Geometry check sheet. Reference: the model listing, model coordinates, mm. Face numbers are marked on the shaded views. A direction names the side the tool comes from. Round coordinates to 2 decimals unless told otherwise and drop trailing zeros. Order: outer loops, then holes, each group sorted by start corner. A loop starts at its lowest first (then second) coordinate and runs counter-clockwise, first axis right, second up.
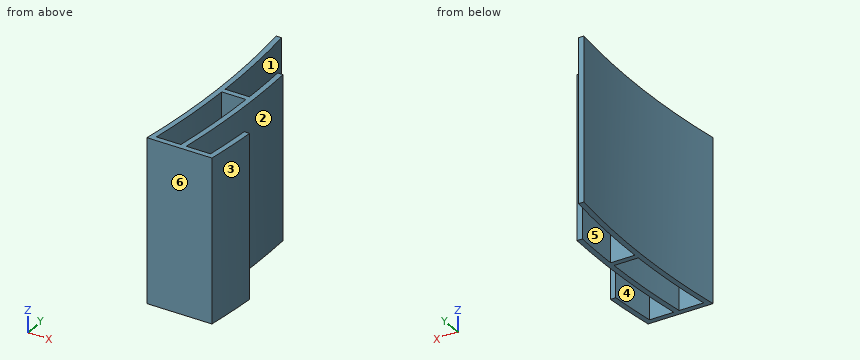
```python
from build123d import *

# Parameters (mm, degrees)
PAD_DEPTH = 60


with BuildPart() as part:
    # Sketch → Pad (new body)
    with BuildSketch(Plane.XY):
        with BuildLine():
            Line((2.414743, -35), (11.414743, -35))
            ThreePointArc((11.414743, -35), (11.263358, -26.246135), (10.865622, -17.5))
            Line((10.865622, -17.5), (12.865622, -17.5))
            ThreePointArc((11.335628, -72), (13.289566, -44.783378), (12.865622, -17.5))
            Line((11.335628, -72), (20.335628, -72))
            ThreePointArc((20.335628, -72), (21.198564, -63.260143), (21.822782, -54.5))
            Line((21.822782, -54.5), (23.822782, -54.5))
            ThreePointArc((22.11492, -74), (23.116177, -64.262903), (23.822782, -54.5))
            Line((22.11492, -74), (-2, -74))
            ThreePointArc((-2, -74), (0.416398, -36), (-2, 2))
            Line((-2, 2), (0.016131, 2))
            ThreePointArc((2.414743, -35), (1.783801, -16.463154), (0.016131, 2))
        make_face()
        with BuildLine():
            Line((2.414743, -37), (11.414743, -37))
            ThreePointArc((9.325722, -72), (10.863864, -54.529463), (11.414743, -37))
            Line((9.325722, -72), (0.263026, -72))
            ThreePointArc((0.263026, -72), (1.847307, -54.531257), (2.414743, -37))
        make_face(mode=Mode.SUBTRACT)
    extrude(amount=PAD_DEPTH)


solid = part.part
```
(1) Sectioned sample at B-B, the plane x = 4.5. Record the cut outline in (y, z).
Returned:
outline: (-74, 0) - (-72, 0) - (-72, 60) - (-74, 60) - close; (-37, 0) - (-35, 0) - (-35, 60) - (-37, 60) - close
(2) Material ranges on line 1 (Y direction, x = 9, z = 52); line 2 (Y direction, x = 14, z = 4.5); line 3 (X direction, y = -36, z = 15), recorded low to high.
Returned:
line 1: y = -74 to -72, -37 to -35
line 2: y = -74 to -72
line 3: x = 0.42 to 13.41
(3) Sectioned sample at A-A, the plane z = 37.5. Record the cut outline in (x, y), and give its area (3 significant figures).
Returned:
outline: (-2, -74) - (22.11, -74) arc R323.94 ccw to (23.82, -54.5) - (21.82, -54.5) arc R321.94 cw to (20.34, -72) - (11.34, -72) arc R313 ccw to (12.87, -17.5) - (10.87, -17.5) arc R311 cw to (11.41, -35) - (2.41, -35) arc R302 ccw to (0.02, 2) - (-2, 2) arc R300 cw to start; hole (0.26, -72) - (9.33, -72) arc R311 ccw to (11.41, -37) - (2.41, -37) arc R302 cw to start
area: 359 mm2
(4) Depth check by flat-ended pin: P1, Ø2.5, axis at x = 6.5, z = 23, coming from the +Y side; P2, Ø4.5, axis at x = 13.5, z = 24, coming from the +Y side; P3, Ø5, axis at x = 8, y = -25, coming from the -Z side; P4, Ø12, axis at y = -38, z = 43.5, coming from the +X side. Enter the tip coordinate at first touch or a pass-through.
Returned:
P1: stops at y = -35
P2: stops at y = -17.5
P3: passes through
P4: stops at x = 13.41
(5) Set-up check for the marked faces 1, 2 and 3: record each of +Z, -Z, +X, -X, +Y, -Y from which the full face is reachable in a straight line by a thin tool's end or side.
Returned:
face 1: +Z, -Z, +Y
face 2: +Z, -Z
face 3: +Z, -Z, +X, -Y
(6) Draft check along Y on the marked faces 4, 5 and 6. Enter one of: released by +Y, released by -Y, zero draft, split by the parting line, or undercut.
Returned:
face 4: released by +Y
face 5: undercut
face 6: released by -Y
(7) Sectioned sample at C-C, the plane y = -59. Record the cut outline in (x, z), and give its area (3 significant figures).
Returned:
outline: (-0.47, 0) - (1.54, 0) - (1.54, 60) - (-0.47, 60) - close; (10.56, 0) - (12.57, 0) - (12.57, 60) - (10.56, 60) - close; (21.53, 0) - (23.53, 0) - (23.53, 60) - (21.53, 60) - close
area: 361 mm2
(8) Sectioned sample at D-D, the plane y = -32. Record the cut outline in (x, z).
Returned:
outline: (0.39, 0) - (2.39, 0) - (2.39, 60) - (0.39, 60) - close; (11.39, 0) - (13.39, 0) - (13.39, 60) - (11.39, 60) - close
